Autodesk Inventor part; units mm, degrees
ref_plane "YZ Plane" through (0, 0, 0) normal (1, 0, 0) x (0, 1, 0)
ref_plane "XZ Plane" through (0, 0, 0) normal (0, 1, 0) x (-1, 0, 0)
ref_plane "XY Plane" through (0, 0, 0) normal (0, 0, 1) x (1, 0, 0)
sketch "Esquisse1" plane through (0, 0, 0) normal (0, 1, 0) x (-1, 0, 0)
  line L0 (-25, -45) -> (-28, -45)
  line L1 (-28, -45) -> (-28, 45)
  line L2 (-28, 45) -> (-25, 45)
  line L3 (-25, 45) -> (-25, -45)
  line L4 (25, 45) -> (28, 45)
  line L5 (28, 45) -> (28, -45)
  line L6 (28, -45) -> (25, -45)
  line L7 (25, -45) -> (25, 45)
  line L8 (-25, 12.5) -> (25, 12.5)
  line L9 (25, 12.5) -> (25, 9.5)
  line L10 (25, 9.5) -> (-25, 9.5)
  line L11 (-25, 9.5) -> (-25, 12.5)
  line L12 (-25, -9.5) -> (25, -9.5)
  line L13 (25, -9.5) -> (25, -12.5)
  line L14 (25, -12.5) -> (-25, -12.5)
  line L15 (-25, -12.5) -> (-25, -9.5)
  point P0 (0, 0)
  dimension "d0" = 50
  dimension "d1" = 3
  dimension "d2" = 3
  dimension "d3" = 3
  dimension "d4" = 3
  dimension "d5" = 25
  dimension "d6" = 90
  dimension "d7" = 25
  dimension "d9" = 45
  dimension "d10" = 12.5
extrude "Extrusion1" add sketch "Esquisse1" along normal blind 40 contours L0 L1 L2 L3 | L3 L12 L7 L14 | L7 L4 L5 L6 | L3 L8 L7 L10
sketch "Esquisse2" plane through (28, 0, 45) normal (1, 0, 0) x (0, 0, -1)
  line L0 (90, 0) -> (90, 40)
  line L1 (0, 0) -> (0, 40)
  circle A0 centre (80, 9.5) radius 6
  line L2 (0, 40) -> (90, 40)
  line L3 (80, 9.5) -> (10, 9.5) construction
  line L4 (10, 9.5) -> (10, 30.5) construction
  line L5 (10, 30.5) -> (80, 30.5) construction
  line L6 (80, 30.5) -> (80, 9.5) construction
  circle A1 centre (10, 30.5) radius 6
  line L7 (0, 0) -> (90, 0)
  line L8 (90, 40) -> (41, 40)
  line L9 (41, 40) -> (41, 20)
  line L10 (41, 20) -> (90, 20)
  line L11 (90, 20) -> (90, 40)
  line L12 (41, 40) -> (21, 40)
  line L13 (21, 40) -> (21, 20) construction
  line L14 (21, 20) -> (41, 20) construction
  line L15 (41, 20) -> (41, 40)
  line L16 (41, 20) -> (21, 40)
  point P0 (45, 0)
  dimension "d14" = 12
  dimension "d21" = 10
  dimension "d22" = 10
  dimension "d23" = 12
  dimension "d24" = 21
  dimension "d25" = 9.5
  dimension "d26" = 40
  dimension "d27" = 20
  dimension "d28" = 20
  dimension "d29" = 21
extrude "Extrusion2" cut sketch "Esquisse2" against normal through all contours L10 L9 L2 L0 | L16 L2 L9 | A0 | A1
sketch "Esquisse4" plane through (-25, 0, 12.5) normal (0, 0, 1) x (1, 0, 0)
  line L0 (50, 28.5) -> (0, 28.5)
  line L1 (0, 0) -> (0, 28.5)
  line L2 (0, 0) -> (50, 0)
  line L3 (0, 0) -> (50, 0)
  line L4 (50, 0) -> (50, 15)
  line L5 (50, 15) -> (0, 15)
  line L6 (0, 15) -> (0, 0)
  line L7 (50, 0) -> (50, 40)
  line L8 (50, 40) -> (53, 40)
  point P0 (25, 0)
  dimension "d33" = 25
extrude "Extrusion3" cut sketch "Esquisse4" against normal through all contours L7 L5 L1 L0
fillet "Congé2" radius 20 2 edges at (26.5, 0, 45) (-26.5, 0, 45)
fillet "Congé3" radius 5 6 edges at (26.5, 40, 45) (-26.5, 40, 45) (26.5, 20, -45) (26.5, 0, -45) (-26.5, 20, -45) (-26.5, 0, -45)
chamfer "Chanfrein1" distance 4 angle 45 4 edges at (-25, 15, 11) (-25, 15, -11) (25, 15, -11) (25, 15, 11)
equation "\"d2\" = d1"
equation "\"d4\" = d3"
equation "\"d23\" = d14"
equation "\"d25\" = -0.5 * d24 + 0.5 * d26"
equation "\"d27\" = 0.5 * d26"
equation "\"d28\" = d27"
properties part number "new_leg_1"
Build history of the part. All positions in model axes, mm. A direction names the side the tool comes from. Coordinates: 2 decimals unless noted, no trailing zeros. Order: outer loops, then holes, each group sorted by start corner. A loop starts at its lowest first (then second) coordinate and runs counter-clockwise, first axis right, second up. Notation, with made-up numbers: (13.5, 78) -> (72.5, 78) arc R19 ccw to (72.5, 115) -> close; hole circle Ø1 at (82.25, 88.25). An arc over 180 degrees is marked (long way). One line per item, written item: value.
(1) Slice it at C-C, the plane y = 30.5. List the corners of the cut face in (x, z).
Checked values:
outline: (-28, 14.5) -> (-25, 14.5) -> (-25, 29) -> (-28, 29) -> close; (-28, 41) -> (-25, 41) -> (-25, 45) -> (-28, 45) -> close; (25, 14.5) -> (28, 14.5) -> (28, 29) -> (25, 29) -> close; (25, 41) -> (28, 41) -> (28, 45) -> (25, 45) -> close
(2) Probe line 1 (Z direction, x = -7.5, y = 5); line 2 (X direction, y = 16, z = -34.5); line 3 (Y direction, x = -27.2, z = -35). List the from-to ranges inside material, lowest first. Write a range as [from, to].
Checked values:
line 1: [-12.5, -9.5], [9.5, 12.5]
line 2: [-28, -25], [25, 28]
line 3: [0, 3.5], [15.5, 20]
(3) Drop flat-ended pins along their axis: pin 1 Ø9.5 at (x, y) = (-9.5, 11) entering from -Z; pin 2 Ø15 at (x, y) = (9.5, 9.5) entering from +Z; pin 3 Ø0.9 at (x, z) = (-4, 10.5) entering from +Y. Give the stop position or say it passes through.
Checked values:
pin 1: z = -12.5
pin 2: z = 12.5
pin 3: y = 15
(4) Mould opens along Z. For faces 1 (the flat face through (0, 15, -11)), 2 (the cylindrical face through (26, 19, -43)), 3 (the cylindrical face through (-26.521, 5.703, 38.986)), 4 (the flat face through (0, 7, 9.5)) say: pulls with the +Z half, pulls with the -Z half, needs draft (parallel to the pull), parting line crosses it, or undercut.
Checked values:
face 1: needs draft
face 2: pulls with the -Z half
face 3: pulls with the +Z half
face 4: undercut
(5) Tool access for faces 5 (the flat face through (0, 7, -12.5)), 6 (the flat face through (27, 40, 32)), 7 (the flat face through (-23, 17, 11)): list every direction of +Z, -Z, +X, -X, +Y, -Y with a clear straight run to the whole face (end or side of a thin tool).
Checked values:
face 5: -Z, +Y, -Y
face 6: +Z, -Z, +X, -X, +Y
face 7: +Z, -Z, +Y
(6) Slice it at B-B, the plane z = 15. List the corners of the cut face in (x, y).
Checked values:
outline: (-28, 0) -> (-25, 0) -> (-25, 31) -> (-28, 31) -> close; (25, 0) -> (28, 0) -> (28, 31) -> (25, 31) -> close
(7) Slice it at A-A, the plane y = 23. List the corners of the cut face in (x, z).
Checked values:
outline: (-28, 7) -> (-25, 7) -> (-25, 45) -> (-28, 45) -> close; (25, 7) -> (28, 7) -> (28, 45) -> (25, 45) -> close
(8) Slice it at D-D, the plane z = -35. List the corners of the cut face in (x, y), plus the area to 3 significant figures.
Checked values:
outline: (-28, 0) -> (-25, 0) -> (-25, 3.5) -> (-28, 3.5) -> close; (-28, 15.5) -> (-25, 15.5) -> (-25, 20) -> (-28, 20) -> close; (25, 0) -> (28, 0) -> (28, 3.5) -> (25, 3.5) -> close; (25, 15.5) -> (28, 15.5) -> (28, 20) -> (25, 20) -> close
area: 48.0 mm2
